Read the model definition and answer for the solid it produces. Units are mm, in the model's axes. Coordinates: 2 decimals unless noted, no trailing zeros. Loops run counter-clockwise (first coordinate to the right, second up) from the corner with the lowest first, then second, coordinate; pieces in that order, holes last.
Q1. Section A-A (x = 0) is taken. Give the vertices of the cut face in (y, z).
Q2. A flat-ended cylindrical pin translates along its axis: P1, Ø7, axis at x = 0, y = -32.85, coming from the -Z side. Find the tip coordinate at first contact, or state that the pin passes through.
Q3. Section D-D (z = 1.1) is taken. Give the vertices of the cut face in (x, y), then the cut area to 3 significant figures.
Q4. Straight lines are drawn through the part: line 1 (Y direction, x = 0, z = 0.65); line 2 (Y direction, x = -2, z = 0.5); line 3 (X direction, y = 33, z = 1.2). For each, find the intervals that lie inside material, in ascending order.
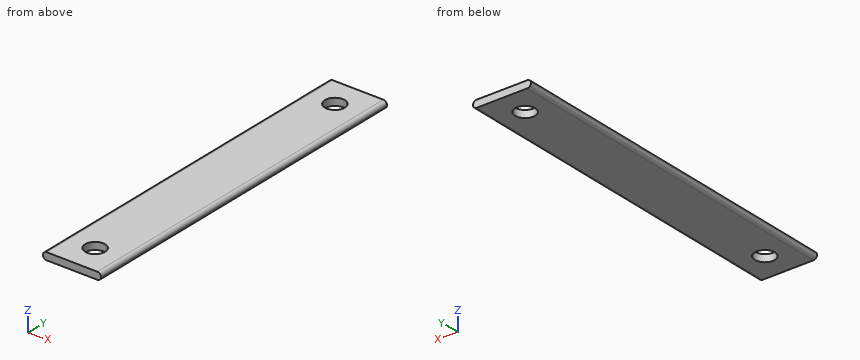
Autodesk Inventor part; units mm, degrees
ref_plane "YZ Plane" through (0, 0, 0) normal (1, 0, 0) x (0, 1, 0)
ref_plane "XZ Plane" through (0, 0, 0) normal (0, 1, 0) x (-1, 0, 0)
ref_plane "XY Plane" through (0, 0, 0) normal (0, 0, 1) x (1, 0, 0)
sketch "Sketch1" plane through (0, 0, 0) normal (0, 0, 1) x (1, 0, 0)
  circle A0 centre (0, 32.85) radius 2.1828
  circle A1 centre (0, -32.85) radius 2.1828
  line L0 (-6.35, -39.2) -> (6.35, -39.2)
  line L1 (6.35, -39.2) -> (6.35, 39.2)
  line L2 (6.35, 39.2) -> (-6.35, 39.2)
  line L3 (-6.35, 39.2) -> (-6.35, -39.2)
  line L4 (-6.35, -39.2) -> (6.35, 39.2) construction
  line L5 (6.35, -39.2) -> (-6.35, 39.2) construction
  point P0 (0, 0)
  dimension "d0" = 4.3656
  dimension "d1" = 4.3656
  dimension "d2" = 65.7
  dimension "d3" = 32.85
  dimension "d4" = 32.85
  dimension "d5" = 12.7
  dimension "d6" = 6.35
extrude "Extrusion1" add sketch "Sketch1" along normal blind 1.5875
fillet "Fillet1" radius 0.7937 4 edges at (-6.35, 0, 0) (-6.35, 0, 1.5875) (6.35, 0, 0) (6.35, 0, 1.5875)
properties part number "Part H"
Numbers:
1. outline: (-39.2, 0) - (-35.03, 0) - (-35.03, 1.59) - (-39.2, 1.59) - close; (-30.67, 0) - (30.67, 0) - (30.67, 1.59) - (-30.67, 1.59) - close; (35.03, 0) - (39.2, 0) - (39.2, 1.59) - (35.03, 1.59) - close
2. P1: stops at z = 0
3. outline: (-6.29, -39.2) - (6.29, -39.2) - (6.29, 39.2) - (-6.29, 39.2) - close; hole circle Ø4.37 at (0, -32.85); hole circle Ø4.37 at (0, 32.85)
3. area: 956 mm2
4. line 1: y = -39.2 to -35.03, -30.67 to 30.67, 35.03 to 39.2
4. line 2: y = -39.2 to -33.72, -31.98 to 31.98, 33.72 to 39.2
4. line 3: x = -6.24 to -2.18, 2.18 to 6.24
